```python
from build123d import *

# Parameters (mm, degrees)
F0_R     = 17.5
F0_W     = 10
F0_H     = 28.6961602334
F0_W_2   = 8
F0_H_2   = 15
F1_DEPTH = 15


# Not quite as in the source:
# - a feature of the source that left no trace in its solid (it failed there, or was rolled back) is left out


with BuildPart() as f1:
    # F0 (on Top) → F1 (new body)
    with BuildSketch(Plane.XY):
        Polygon((122.6644553625, 14.977986814), (122.6644553625, 39.977986814), (-32.3355446375, 39.977986814), (-32.3355446375, 14.977986814), (-29.8321247846, 14.977986814), (-19.8321247846, 14.977986814), (-9.8321247846, 14.977986814), (-1.8321247846, 14.977986814), (8.1678752154, 14.977986814), (22.2149824233, 14.977986814), align=None)
        with BuildLine():
            ThreePointArc((122.6644553625, 14.977986814), (190.356197439, 27.477986814), (122.6644553625, 39.977986814))
            Line((122.6644553625, 39.977986814), (122.6644553625, 14.977986814))
        make_face()
        with Locations((155.356197439, 27.477986814)):
            Circle(F0_R, mode=Mode.SUBTRACT)
        with Locations((-24.8321247846, 0.6299066973)):
            Rectangle(F0_W, F0_H)
        with Locations((-5.8321247846, 7.477986814)):
            Rectangle(F0_W_2, F0_H_2)
        Polygon((15.1678752154, 0), (22.2149824233, 14.977986814), (8.1678752154, 14.977986814), align=None)
    extrude(amount=F1_DEPTH)


solid = f1.part
```
Geometry: final body of the model. Coordinates: model frame, mm. A direction names the side the tool comes from. Coordinates: 2 decimals unless noted, no trailing zeros. Order: outer loops, then holes, each group sorted by start corner. A loop starts at its lowest first (then second) coordinate and runs counter-clockwise, first axis right, second up. Notation, with made-up numbers: (-27.5, 21) - (8.5, 21) arc R29 cw to (8.5, 51) - close; hole circle Ø10 at (66.25, 8.5). An arc over 180 degrees is marked (long way). Write each question's results on one line, items separated by ' | '.
(1) Line query: line 1 (X direction, y = 7, z = 5.5); line 2 (X direction, y = 8.5, z = 3); line 3 (X direction, y = 27.5, z = 5.5). Output: solid intervals per line, ascending. Write a range as [from, to].
Values found:
line 1: x = [-29.83, -19.83], [-9.83, -1.83], [11.9, 18.46], [126.97, 183.74] | line 2: x = [-29.83, -19.83], [-9.83, -1.83], [11.2, 19.17], [125.95, 184.76] | line 3: x = [-32.34, 137.86], [172.86, 190.36]
(2) Mould query, pull axis Y, two halves, no side actions, for faces 4 (the face through (-6, -0.022, 7)), 5 (the face through (-9.832, 7, 7)), 6 (the face through (141.47, 16.83, 7.4)). Classes: +Y half, -Y half, draft (parallel to the pull), parting line (faces both ways), or undercut.
Values found:
face 4: -Y half | face 5: draft | face 6: undercut
(3) Set-up query: faces 1 (the face through (46, 39.978, 7)), 2 (the face through (-29.832, 0, 7)), 3 (the face through (11.62, 7.59, 7.4)). Return all of +Z, -Z, +X, -X, +Y, -Y with unobstructed straight access to the full face (end or side cutting, diameter ignored); none if empty.
Values found:
face 1: +Z, -Z, -X, +Y | face 2: +Z, -Z, -X, -Y | face 3: +Z, -Z, -Y
(4) Section query A-A, the plane y = 38. Return the cut outline in (x, z), plus the area to 3 significant figures.
Values found:
outline: (-32.34, 0) - (141.37, 0) - (141.37, 15) - (-32.34, 15) - close; (169.34, 0) - (188.74, 0) - (188.74, 15) - (169.34, 15) - close | area: 2,900 mm²
(5) Section query C-C, the plane x = 99. Return the cut outline in (y, z), plus the area to 3 significant figures.
Values found:
outline: (14.98, 0) - (39.98, 0) - (39.98, 15) - (14.98, 15) - close | area: 375 mm²
(6) Section query D-D, the plane y = 51. Return the cut outline in (x, z), plus the area to 3 significant figures.
Values found:
outline: (129.44, 0) - (181.27, 0) - (181.27, 15) - (129.44, 15) - close | area: 778 mm²
(7) Section query B-B, the plane z = 7.25. Return the cut outline in (x, y), plus the area to 3 significant figures.
Values found:
outline: (-32.34, 14.98) - (-29.83, 14.98) - (-29.83, -13.72) - (-19.83, -13.72) - (-19.83, 14.98) - (-9.83, 14.98) - (-9.83, -0.02) - (-1.83, -0.02) - (-1.83, 14.98) - (8.17, 14.98) - (15.17, 0) - (22.21, 14.98) - (122.66, 14.98) arc R35 ccw (long way) to (122.66, 39.98) - (-32.34, 39.98) - close; hole circle Ø35 at (155.36, 27.48) | area: 7,230 mm²
(8) First-contact query: pin 1 Ø7.5 at (y, z) = (6.5, 7) entering from +X; pin 2 Ø8 at (x, z) = (-15, 7) entering from -Y; pin 3 Ø7.5 at (y, z) = (1, 7.5) entering from -X; pin 4 Ø1 at (x, y) = (-1, 13) entering from -Z. Flat tips, straight axial feed; report the tip coordinate or a pass-through.
Values found:
pin 1: stops at x = 185.82 | pin 2: stops at y = 14.98 | pin 3: stops at x = -29.83 | pin 4: passes through
